Geometry: final body of the model. Coordinates: model frame, mm. Face numbers are marked on the shaded views. Give positions to 0.01 mm unless a question says otherwise; leave off trailing zeros. Loops run counter-clockwise (first coordinate to the right, second up) from the corner with the lowest first, then second, coordinate; pieces in that order, holes last.
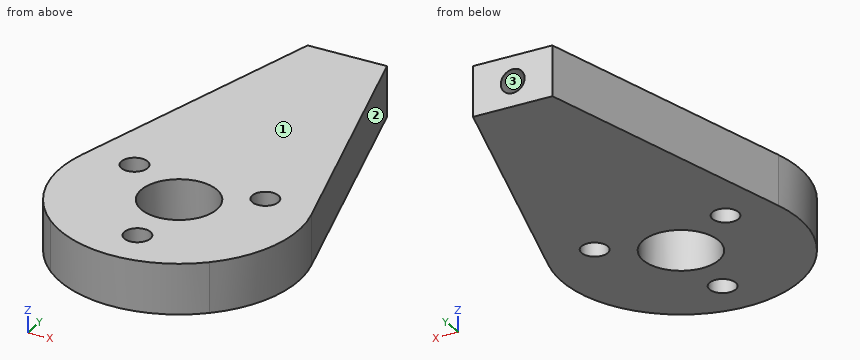
```python
from build123d import *

# Parameters (mm, degrees)
BASE_DEPTH           = 3.175
BOSS_EXTRUDE1_DEPTH  = 6.35
SKETCH2_R            = 4.77266
SHAFT_AND_BOLT_DEPTH = 7.35
SKETCH5_R            = 1.5
CUT_EXTRUDE1_DEPTH   = 14
SKETCH6_R            = 1.65
CUT_EXTRUDE2_DEPTH   = 7.35


with BuildPart() as part:
    # Sketch1 → Base (new body, symmetric)
    with BuildSketch(Plane.XY):
        with BuildLine():
            Line((-5, 38.38), (-14.46282813, 3.978266268))
            ThreePointArc((-14.46282813, 3.978266268), (-14.389347628, -4.236351595), (-10, -11.180339887))
            Line((-10, -11.180339887), (10, -11.180339887))
            ThreePointArc((10, -11.180339887), (14.389347628, -4.236351595), (14.46282813, 3.978266268))
            Line((14.46282813, 3.978266268), (5, 38.38))
            Line((5, 38.38), (-5, 38.38))
        make_face()
    extrude(amount=BASE_DEPTH, both=True)

    # Sketch7 → Boss-Extrude1 (add)
    with BuildSketch(Plane.XY.offset(3.175)):
        with BuildLine():
            Line((-10, -11.180339887), (10, -11.180339887))
            ThreePointArc((10, -11.180339887), (0, -15), (-10, -11.180339887))
        make_face()
    extrude(amount=-BOSS_EXTRUDE1_DEPTH)

    # Sketch2 → Shaft and Bolt (cut, through all)
    with BuildSketch(Plane.XY.offset(3.175)):
        Circle(SKETCH2_R)
    extrude(amount=-SHAFT_AND_BOLT_DEPTH, mode=Mode.SUBTRACT)

    # Sketch5 → Cut-Extrude1 (cut)
    with BuildSketch(Plane(origin=(0, 38.38, 0), x_dir=(1, 0, 0), z_dir=(0, 1, 0))):
        Circle(SKETCH5_R)
    extrude(amount=-CUT_EXTRUDE1_DEPTH, mode=Mode.SUBTRACT)

    # Sketch6 → Cut-Extrude2 (cut, through all)
    with BuildSketch(Plane.XY.offset(3.175)):
        with Locations((0, -9.5125)):
            Circle(SKETCH6_R)
        with Locations((-8.238066653, 4.75625)):
            Circle(SKETCH6_R)
        with Locations((8.238066653, 4.75625)):
            Circle(SKETCH6_R)
    extrude(amount=-CUT_EXTRUDE2_DEPTH, mode=Mode.SUBTRACT)


solid = part.part
```
Q1. Section query D-D, the plane y = 26.5. Return loops of the section in (x, z) (3 decimals).
Q2. Section query B-B, the plane x = 0. Return loops of the section in (y, z) (1 decimal), and give its area (3 significant figures).
Q3. Mould query, pull axis Z, two halves, no side actions, for the marked faces 1, 2 and 3. Classes: +Z half, -Z half, draft (parallel to the pull), parting line (faces both ways), or undercut.
Q4. Material intervals for probe 1 along Y at (x, z) = (0, -1.25); probe 2 along Y at (x, z) = (-1.5, 0.75); probe 3 along Z at (x, y) = (0, 33) (3 decimals), sorted ascending.
Q5. Section query C-C, the plane z = 0. Return loops of the section in (x, y), and give its area (3 significant figures).
Q6. Pin query (flat end, axial travel): pin 1 Ø1.5 at (x, z) = (-0.5, 0) entering from +Y; pin 2 Ø2 at (y, z) = (-4, 0.5) entering from -X; pin 3 Ø1.5 at (y, z) = (16, -2) entering from +X; pin 4 Ø2 at (x, y) = (0.5, 3.5) entering from -Z. Return the tip coordinate at first contact, or that it passes through.
Q7. Section query A-A, the plane y = 0. Return loops of the section in (x, z) (3 decimals).
Resolved:
1. outline: (-8.268, -3.175) - (8.268, -3.175) - (8.268, 3.175) - (-8.268, 3.175) - close; hole circle Ø3 at (0, 0)
2. outline: (-15, -3.2) - (-11.2, -3.2) - (-11.2, 3.2) - (-15, 3.2) - close; (-7.9, -3.2) - (-4.8, -3.2) - (-4.8, 3.2) - (-7.9, 3.2) - close; (4.8, -3.2) - (38.4, -3.2) - (38.4, -1.5) - (24.4, -1.5) - (24.4, 1.5) - (38.4, 1.5) - (38.4, 3.2) - (4.8, 3.2) - close
2. area: 215 mm2
3. face 1: +Z half
3. face 2: draft
3. face 3: undercut
4. probe 1: y = -15 to -11.16, -7.86 to -4.77, 4.77 to 24.38
4. probe 2: y = -14.92 to -10.2, -8.83 to -4.53, 4.53 to 38.38
4. probe 3: z = -3.175 to -1.5, 1.5 to 3.175
5. outline: (-14.46, 3.98) arc R15 ccw (long way) to (14.46, 3.98) - (5, 38.38) - (1.5, 38.38) - (1.5, 24.38) - (-1.5, 24.38) - (-1.5, 38.38) - (-5, 38.38) - close; hole circle Ø3.3 at (-8.24, 4.76); hole circle Ø9.55 at (0, 0); hole circle Ø3.3 at (0, -9.51); hole circle Ø3.3 at (8.24, 4.76)
5. area: 1,000 mm2
6. pin 1: stops at y = 24.38
6. pin 2: stops at x = -14.7
6. pin 3: stops at x = 11.36
6. pin 4: passes through
7. outline: (-15, -3.175) - (-4.773, -3.175) - (-4.773, 3.175) - (-15, 3.175) - close; (4.773, -3.175) - (15, -3.175) - (15, 3.175) - (4.773, 3.175) - close
